Part model, mm, in its own coordinate system. Give positions to 0.01 mm unless a question says otherwise; leave off trailing zeros. Order: outer loops, then holes, each group sorted by start corner. A loop starts at its lowest first (then second) coordinate and runs counter-clockwise, first axis right, second up. Notation, with made-up numbers: (-24, 50) - (-1, 50) arc R19 cw to (-1, 86) - close; hole circle Ø7 at (50, 16). An arc over 180 degrees is marked (long way). Use one line per item in the form item = value. Start each with the question number.
1. Band-saw the part on C-C, the plane x = 5. List the corners of the cut face in (y, z), plus the area to 3 significant figures.
2. Band-saw the part on B-B, the plane y = 8.5. State how many separate pieces and enclosed holes the cut face has, plus the area to 3 significant figures.
3. Drill centre lines: line 1 (Z direction, x = 5, y = 3.75); line 2 (X direction, y = 8.7, z = -17.5); line 3 (Y direction, x = 10, z = -7.5). Where is each one in solid material? Low to high.
4. Pull direction X, two halves, no side cores. Call faces 1 (the face through (5.07, 9.62, -19.15)), 2 (the face through (30.054, 4.475, -18.131)): +X half, -X half, draft (parallel to the pull), parting line (faces both ways), or undercut.
5. Band-saw the part on A-A, the plane z = -22.5. List the corners of the cut face in (x, y).
6. Band-saw the part on D-D, the plane x = 10. List the corners of the cut face in (y, z), plus the area to 3 significant figures.
from build123d import *

# Parameters (mm, degrees)
ESQUISSE1_W             = 25
ESQUISSE1_H             = 12
BOSS_EXTRU_1_DEPTH      = 40
ESQUISSE2_R             = 1.65
ENL_V_MAT_EXTRU_1_DEPTH = 49.672374095
ESQUISSE3_R             = 1.65
ENL_V_MAT_EXTRU_2_DEPTH = 40
ESQUISSE4_R             = 1.65
ENL_V_MAT_EXTRU_3_DEPTH = 40


with BuildPart() as part:
    # Esquisse1 → Boss.-Extru.1 (new body)
    with BuildSketch(Plane(origin=(0, 0, 0), x_dir=(0, 0, -1), z_dir=(1, 0, 0))):
        with Locations((12.5, 6)):
            Rectangle(ESQUISSE1_W, ESQUISSE1_H)
    extrude(amount=BOSS_EXTRU_1_DEPTH)

    # Esquisse2 → Enlèv. mat.-Extru.1 (cut, through all)
    with BuildSketch(Plane(origin=(0, 12, 0), x_dir=(1, 0, 0), z_dir=(0, 1, 0))):
        with Locations(Location((5, 17.5, 0), (0, 0, 270))):
            Circle(ESQUISSE2_R)
        with Locations(Location((15, 17.5, 0), (0, 0, 270))):
            Circle(ESQUISSE2_R)
        with Locations(Location((25, 17.5, 0), (0, 0, 270))):
            Circle(ESQUISSE2_R)
        with Locations(Location((35, 17.5, 0), (0, 0, 270))):
            Circle(ESQUISSE2_R)
        with Locations(Location((5, 7.5, 0), (0, 0, 270))):
            Circle(ESQUISSE2_R)
        with Locations(Location((15, 7.5, 0), (0, 0, 270))):
            Circle(ESQUISSE2_R)
        with Locations(Location((35, 7.5, 0), (0, 0, 270))):
            Circle(ESQUISSE2_R)
        with Locations(Location((25, 7.5, 0), (0, 0, 270))):
            Circle(ESQUISSE2_R)
    extrude(amount=-ENL_V_MAT_EXTRU_1_DEPTH, mode=Mode.SUBTRACT)

    # Esquisse3 → Enlèv. mat.-Extru.2 (cut)
    with BuildSketch(Plane.XY):
        with Locations((5, 6)):
            Circle(ESQUISSE3_R)
        with Locations((15, 6)):
            Circle(ESQUISSE3_R)
        with Locations((25, 6)):
            Circle(ESQUISSE3_R)
        with Locations((35, 6)):
            Circle(ESQUISSE3_R)
    extrude(amount=-ENL_V_MAT_EXTRU_2_DEPTH, mode=Mode.SUBTRACT)

    # Esquisse4 → Enlèv. mat.-Extru.3 (cut)
    with BuildSketch(Plane(origin=(40, 0, 0), x_dir=(0, 0, -1), z_dir=(1, 0, 0))):
        with Locations(Location((17.5, 6, 0), (0, 0, 315))):
            Circle(ESQUISSE4_R)
        with Locations(Location((7.5, 6, 0), (0, 0, 315))):
            Circle(ESQUISSE4_R)
    extrude(amount=-ENL_V_MAT_EXTRU_3_DEPTH, mode=Mode.SUBTRACT)


solid = part.part
From the geometry:
q1.outline = (0, -25) - (4.35, -25) - (4.35, -19.15) - (0, -19.15) - close; (0, -15.85) - (4.35, -15.85) - (4.35, -9.15) - (0, -9.15) - close; (0, -5.85) - (4.35, -5.85) - (4.35, 0) - (0, 0) - close; (7.65, -25) - (12, -25) - (12, -19.15) - (7.65, -19.15) - close; (7.65, -15.85) - (12, -15.85) - (12, -9.15) - (7.65, -9.15) - close; (7.65, -5.85) - (12, -5.85) - (12, 0) - (7.65, 0) - close
q1.area = 160 mm²
q2.separate_pieces = 1
q2.enclosed_holes = 8
q2.area = 932 mm²
q3.line_1 = -25 to -19.15, -15.85 to -9.15, -5.85 to 0
q3.line_2 = 0 to 3.35, 6.65 to 13.35, 16.65 to 23.35, 26.65 to 33.35, 36.65 to 40
q3.line_3 = 0 to 4.35, 7.65 to 12
q4.face_1 = undercut
q4.face_2 = draft
q5.outline = (0, 0) - (40, 0) - (40, 12) - (0, 12) - close; hole circle Ø3.3 at (5, 6); hole circle Ø3.3 at (15, 6); hole circle Ø3.3 at (25, 6); hole circle Ø3.3 at (35, 6)
q6.outline = (0, -25) - (12, -25) - (12, 0) - (0, 0) - close; hole circle Ø3.3 at (6, -17.5); hole circle Ø3.3 at (6, -7.5)
q6.area = 283 mm²
